Work out the finished part from the listing and answer in its coordinate system (mm). A direction names the side the tool comes from. Coordinates: 2 decimals unless noted, no trailing zeros. Write each loop counter-clockwise with the first axis right and the second up, starting at its lowest first coordinate (ties: lowest second). Pieces come first, ordered by that corner, then holes. Notation, with made-up numbers: (-22, 29) - (33, 29) arc R33 ccw to (33, 58) - close; hole circle Ø10 at (22.5, -29.5). An arc over 180 degrees is marked (long way). One line per item, written item: value.
```python
from build123d import *

# Parameters (mm, degrees)
SKETCH_1_W          = 40
SKETCH_1_H          = 20
EXTRUDE_1_DEPTH     = 6
SKETCH_2_W          = 40
SKETCH_2_H          = 32.5
EXTRUDE_2_DEPTH     = 35
CUT_EXTRUDE_1_DEPTH = 13
CUT_EXTRUDE_2_DEPTH = 2
SKETCH_6_W          = 40
SKETCH_6_H          = 41
CUT_EXTRUDE_3_DEPTH = 5
SKETCH_8_R          = 1.7
CUT_EXTRUDE_4_DEPTH = 49.79805324
SKETCH_9_W          = 40
SKETCH_9_H          = 12.5
SKETCH_9_H_2        = 8
CUT_EXTRUDE_5_DEPTH = 41
CUT_EXTRUDE_6_DEPTH = 2
SKETCH_11_R         = 3.2
CUT_EXTRUDE_7_DEPTH = 2.8
SKETCH_12_W         = 0.4
SKETCH_12_H         = 41
CUT_EXTRUDE_8_DEPTH = 5
SKETCH_13_W         = 8
SKETCH_13_H         = 1
CUT_EXTRUDE_9_DEPTH = 2


with BuildPart() as part:
    # Эскиз1 → Бобышка-Вытянуть1 (new body)
    with BuildSketch(Plane.XY):
        Rectangle(SKETCH_1_W, SKETCH_1_H)
    extrude(amount=EXTRUDE_1_DEPTH)

    # Эскиз2 → Бобышка-Вытянуть2 (add)
    with BuildSketch(Plane(origin=(0, 0, 0), x_dir=(-1, 0, 0), z_dir=(0, 0, -1))):
        with Locations((0, 6.25)):
            Rectangle(SKETCH_2_W, SKETCH_2_H)
    extrude(amount=EXTRUDE_2_DEPTH)

    # Эскиз3 → Вырез-Вытянуть1 (cut)
    with BuildSketch(Plane.XZ.offset(10)):
        Polygon((-7, 6), (-7, -1), (-9, -1), (-9, -23), (-6.5, -26), (-6.5, -33), (-4.5, -33), (-4.5, -35), (4.5, -35), (4.5, -33), (6.5, -33), (6.5, -26), (9, -23), (9, -1), (7, -1), (7, 6), align=None)
    extrude(amount=-CUT_EXTRUDE_1_DEPTH, mode=Mode.SUBTRACT)

    # Эскиз5 → Вырез-Вытянуть2 (cut)
    with BuildSketch(Plane.XZ.offset(-3)):
        Polygon((-9, -1), (9, -1), (9, -23), (6.5, -26), (6.5, -33), (-6.5, -33), (-6.5, -26), (-9, -23), align=None)
    extrude(amount=-CUT_EXTRUDE_2_DEPTH, mode=Mode.SUBTRACT)

    # Эскиз6 → Вырез-Вытянуть3 (cut)
    with BuildSketch(Plane.XZ.offset(10)):
        with Locations((0, -14.5)):
            Rectangle(SKETCH_6_W, SKETCH_6_H)
    extrude(amount=-CUT_EXTRUDE_3_DEPTH, mode=Mode.SUBTRACT)

    # Эскиз8 → Вырез-Вытянуть4 (cut, through all)
    with BuildSketch(Plane.XZ.offset(5)):
        with Locations((12, -26)):
            Circle(SKETCH_8_R)
        with Locations((14.5, -6)):
            Circle(SKETCH_8_R)
        with Locations(Location((-12, -26, 0), (0, 0, 180))):
            Circle(SKETCH_8_R)
        with Locations(Location((-14.5, -6, 0), (0, 0, 180))):
            Circle(SKETCH_8_R)
    extrude(amount=-CUT_EXTRUDE_4_DEPTH, mode=Mode.SUBTRACT)

    # Эскиз9 → Вырез-Вытянуть5 (cut)
    with BuildSketch(Plane.XY.offset(6)):
        with Locations((0, 16.25)):
            Rectangle(SKETCH_9_W, SKETCH_9_H)
        with Locations((0, -1)):
            Rectangle(SKETCH_9_W, SKETCH_9_H_2)
    extrude(amount=-CUT_EXTRUDE_5_DEPTH, mode=Mode.SUBTRACT)

    # Эскиз10 → Вырез-Вытянуть6 (cut)
    with BuildSketch(Plane.XZ.offset(-3)):
        Polygon((-20, 6), (-6.4, 6), (-6.4, -1), (-4, -33), (-4, -35), (-20, -35), align=None)
    cut_extrude_6 = extrude(amount=-CUT_EXTRUDE_6_DEPTH, mode=Mode.SUBTRACT)

    # Зеркальное отражение1: Вырез-Вытянуть6 across plane
    add(cut_extrude_6.mirror(Plane(origin=(0, 0, 0), x_dir=(0, 0, 1), z_dir=(1, 0, 0))), mode=Mode.SUBTRACT)

    # Эскиз11 → Вырез-Вытянуть7 (cut)
    with BuildSketch(Plane(origin=(0, 10, 0), x_dir=(1, 0, 0), z_dir=(0, 1, 0))):
        with Locations(Location((14.5, 6, 0), (0, 0, 180))):
            Circle(SKETCH_11_R)
        with Locations((-14.5, 6)):
            Circle(SKETCH_11_R)
        Polygon((-12, 29.233161507), (-14.8, 27.616580754), (-14.8, 24.383419246), (-12, 22.766838493), (-9.2, 24.383419246), (-9.2, 27.616580754), align=None)
        Polygon((9.2, 27.616580754), (12, 29.233161507), (14.8, 27.616580754), (14.8, 24.383419246), (12, 22.766838493), (9.2, 24.383419246), align=None)
    extrude(amount=-CUT_EXTRUDE_7_DEPTH, mode=Mode.SUBTRACT)

    # Эскиз12 → Вырез-Вытянуть8 (cut)
    with BuildSketch(Plane(origin=(0, 10, 0), x_dir=(1, 0, 0), z_dir=(0, 1, 0))):
        with Locations((-19.8, 14.5)):
            Rectangle(SKETCH_12_W, SKETCH_12_H)
        with Locations((19.8, 14.5)):
            Rectangle(SKETCH_12_W, SKETCH_12_H)
    extrude(amount=-CUT_EXTRUDE_8_DEPTH, mode=Mode.SUBTRACT)

    # Эскиз13 → Вырез-Вытянуть9 (cut)
    with BuildSketch(Plane(origin=(0, 0, -35), x_dir=(-1, 0, 0), z_dir=(0, 0, -1))):
        with Locations((0, 3.5)):
            Rectangle(SKETCH_13_W, SKETCH_13_H)
    extrude(amount=-CUT_EXTRUDE_9_DEPTH, mode=Mode.SUBTRACT)


solid = part.part
```
Item 1: Section B-B, the plane y = 6 is taken. Determine the outline of the cut face in (x, z).
Evaluation:
outline: (-19.6, -35) - (19.6, -35) - (19.6, 6) - (-19.6, 6) - close; hole circle Ø3.4 at (-14.5, -6); hole circle Ø3.4 at (-12, -26); hole circle Ø3.4 at (12, -26); hole circle Ø3.4 at (14.5, -6)
Item 2: Given pin 1 (1.6 mm diameter, centred on y = 3.5, z = 3, fed in from -X); pin 2 (4 mm diameter, centred on x = -14.5, z = -6, fed in from +Y); pin 3 (0.8 mm diameter, centred on y = 4.5, z = -34, fed in from -X), each flat-ended and moving along its own axis, determine where each tip first touches the part or whether it passes through.
Evaluation:
pin 1: stops at x = -6.4
pin 2: stops at y = 7.2
pin 3: stops at x = -4
Item 3: Which of the six approach directions +Z, -Z, +X, -X, +Y, -Y give full straight-line access (tool end or side, diameter ignored) to faces 1 (the face through (0, 4, -1)), 2 (the face through (-15.3, 6.1, -4.5)), 3 (the face through (-13.38, 8.62, -28.436))?
Evaluation:
face 1: +X, -X, -Y
face 2: +Y, -Y
face 3: +Y
Item 4: Section C-C, the plane z = -6 is taken. Determine the outline of the cut face in (x, y), then the cut area to 3 significant figures.
Evaluation:
outline: (-19.6, 5) - (-16.2, 5) - (-16.2, 7.2) - (-17.7, 7.2) - (-17.7, 10) - (-19.6, 10) - close; (-12.8, 5) - (12.8, 5) - (12.8, 7.2) - (11.3, 7.2) - (11.3, 10) - (-11.3, 10) - (-11.3, 7.2) - (-12.8, 7.2) - close; (16.2, 5) - (19.6, 5) - (19.6, 10) - (17.7, 10) - (17.7, 7.2) - (16.2, 7.2) - close
area: 145 mm2
Item 5: Section D-D, the plane x = -2.5 is taken. Determine the outline of the cut face in (y, z).
Evaluation:
outline: (3, -1) - (5, -1) - (5, -33) - (4, -33) - (4, -35) - (10, -35) - (10, 6) - (3, 6) - close
Item 6: Section A-A, the plane z = -26 is taken. Determine the outline of the cut face in (x, y), then the cut area to 3 significant figures.
Evaluation:
outline: (-19.6, 5) - (-13.7, 5) - (-13.7, 7.2) - (-14.8, 7.2) - (-14.8, 10) - (-19.6, 10) - close; (-10.3, 5) - (10.3, 5) - (10.3, 7.2) - (9.2, 7.2) - (9.2, 10) - (-9.2, 10) - (-9.2, 7.2) - (-10.3, 7.2) - close; (13.7, 5) - (19.6, 5) - (19.6, 10) - (14.8, 10) - (14.8, 7.2) - (13.7, 7.2) - close
area: 150 mm2
Item 7: Consider probe 1 along Z at (x, y) = (-12, 5.85); probe 2 along Z at (x, y) = (14.5, 6.4); probe 3 along X at (y, z) = (9.5, -7). Determine where each line is inside the solid, lowest interval first.
Evaluation:
probe 1: z = -35 to -27.7, -24.3 to 6
probe 2: z = -35 to -7.7, -4.3 to 6
probe 3: x = -19.6 to -17.54, -11.46 to 11.46, 17.54 to 19.6
Item 8: Determine the mould class of faces 4 (the face through (0, 7, 6)), 5 (the face through (-0.1, 4.5, -33)), 6 (the face through (0, 4, -34)) for opening direction Z: +Z half, -Z half, draft (parallel to the pull), parting line (faces both ways), or undercut.
Evaluation:
face 4: +Z half
face 5: undercut
face 6: draft
